Check sheet for the modelled part. Datum: model origin and axes. Units: mm. A direction names the side the tool comes from. Coordinates: 2 decimals unless noted, no trailing zeros. Loops run counter-clockwise (first coordinate to the right, second up) from the corner with the lowest first, then second, coordinate; pieces in that order, holes last.
```python
from build123d import *

# Parameters (mm, degrees)
BOX073_W     = 7
BOX073_H     = 6
BOX073_DEPTH = 1
BOX072_W     = 8
BOX072_H     = 7
BOX072_DEPTH = 2
BOX071_W     = 7
BOX071_H     = 6
BOX071_DEPTH = 3


with BuildPart() as box073:
    # Box073 → Box073 (new body)
    with BuildSketch(Plane(origin=(11.5, 28.75, 18.6), x_dir=(1, 0, 0), z_dir=(0, 0, 1))):
        with Locations((3.5, 3)):
            Rectangle(BOX073_W, BOX073_H)
    extrude(amount=BOX073_DEPTH)


with BuildPart() as box072:
    # Box072 → Box072 (new body)
    with BuildSketch(Plane(origin=(11, 28.25, 18.6), x_dir=(1, 0, 0), z_dir=(0, 0, 1))):
        with Locations((4, 3.5)):
            Rectangle(BOX072_W, BOX072_H)
    extrude(amount=BOX072_DEPTH)


with BuildPart() as cut009:
    # Box071 → Box071 (new body)
    with BuildSketch(Plane(origin=(11.5, 28.75, 20.6), x_dir=(1, 0, 0), z_dir=(0, 0, 1))):
        with Locations((3.5, 3)):
            Rectangle(BOX071_W, BOX071_H)
    extrude(amount=BOX071_DEPTH)

    # Fusion024: union Box072
    add(box072.part)

    # Cut009: cut Box073
    add(box073.part, mode=Mode.SUBTRACT)


solid = cut009.part
```
1) Set-up check for faces 4 (the flat face through (11.5, 32, 22)), 5 (the flat face through (11.5, 32, 19)), 6 (the flat face through (15, 34.75, 22)): record each of +Z, -Z, +X, -X, +Y, -Y from which the full face is reachable in a straight line by a thin tool's end or side.
Answer sheet:
face 4: +Z, -X, +Y, -Y
face 5: -Z
face 6: +Z, +X, -X, +Y
2) Depth check by flat-ended pin: pin 1 (0.9 mm diameter, centred on y = 31, z = 21.5, fed in from +X); pin 2 (2.5 mm diameter, centred on x = 16.5, z = 22.5, fed in from +Y); pin 3 (1.5 mm diameter, centred on x = 13.5, z = 22.5, fed in from -Y). Enter the tip coordinate at first touch or a pass-through.
Answer sheet:
pin 1: stops at x = 18.5
pin 2: stops at y = 34.75
pin 3: stops at y = 28.75
3) Scan lines: line 1 (Y direction, x = 12.5, z = 19.5); line 2 (X direction, y = 30.25, z = 18.9); line 3 (Z direction, x = 14.5, y = 30.5). Record each from-to range of solid material in increasing order.
Answer sheet:
line 1: y = 28.25 to 28.75, 34.75 to 35.25
line 2: x = 11 to 11.5, 18.5 to 19
line 3: z = 19.6 to 23.6
4) Section check C-C on z = 21.9. Enter the section's corners in (x, y).
Answer sheet:
outline: (11.5, 28.75) - (18.5, 28.75) - (18.5, 34.75) - (11.5, 34.75) - close
5) Section check A-A on x = 13.75. Enter the section's corners in (y, z), plus the area to 3 significant figures.
Answer sheet:
outline: (28.25, 18.6) - (28.75, 18.6) - (28.75, 19.6) - (34.75, 19.6) - (34.75, 18.6) - (35.25, 18.6) - (35.25, 20.6) - (34.75, 20.6) - (34.75, 23.6) - (28.75, 23.6) - (28.75, 20.6) - (28.25, 20.6) - close
area: 26.0 mm2
6) Mould release check, pull along X, two halves, no side actions. Record for faces 1 (the flat face through (15, 32, 23.6)), 2 (the flat face through (18.5, 32, 22)), 3 (the flat face through (15, 32, 19.6)): +X half, -X half, draft (parallel to the pull), parting line (faces both ways), or undercut.
Answer sheet:
face 1: draft
face 2: +X half
face 3: undercut
7) Section check B-B on y = 29.5. Enter the section's corners in (x, z), plus the area to 3 significant figures.
Answer sheet:
outline: (11, 18.6) - (11.5, 18.6) - (11.5, 19.6) - (18.5, 19.6) - (18.5, 18.6) - (19, 18.6) - (19, 20.6) - (18.5, 20.6) - (18.5, 23.6) - (11.5, 23.6) - (11.5, 20.6) - (11, 20.6) - close
area: 30.0 mm2
